Can you work these out from the model? Positions are in its coordinate system, mm. Face numbers are marked on the shaded views. A direction names the side the tool comes from. Round coordinates to 2 decimals unless told otherwise and drop trailing zeros. Loops run counter-clockwise (first coordinate to the right, second up) from the corner with the lowest first, then second, coordinate; pieces in that order, holes last. Notation, with made-up numbers: (50, -28.5) -> (89, -28.5) arc R20 ccw to (89, 10.5) -> close; hole circle Ø9 at (-20.5, 76). An arc over 180 degrees is marked (long way). Answer as a JSON object with one key per item and string values.
```python
from build123d import *

# Parameters (mm, degrees)
SKETCH1_R           = 57.5
BOSS_EXTRUDE1_DEPTH = 18
SKETCH2_R           = 7.5
CUT_EXTRUDE1_DEPTH  = 84.285653026
SKETCH3_R           = 8.629374231
CUT_EXTRUDE2_DEPTH  = 15.116019
CIRPATTERN1_START   = 2.883980854
CIRPATTERN1_DEPTH   = 15.116019146


# Read off the part's stored shape, not the designer's step: CirPattern1
with BuildPart() as part:
    # Sketch1 → Boss-Extrude1 (new body)
    with BuildSketch(Plane(origin=(0, 0, 0), x_dir=(1, 0, 0), z_dir=(0, 1, 0))):
        with Locations(Location((0, 0, 0), (0, 0, 270))):
            Circle(SKETCH1_R)
    extrude(amount=BOSS_EXTRUDE1_DEPTH)

    # Sketch2 → Cut-Extrude1 (cut, through all)
    with BuildSketch(Plane(origin=(0, 0, 0), x_dir=(1, 0, 0), z_dir=(0, 1, 0))):
        with Locations(Location((0, 0, 0), (0, 0, 270))):
            Circle(SKETCH2_R)
    extrude(amount=CUT_EXTRUDE1_DEPTH, mode=Mode.SUBTRACT)

    # Sketch3 → Cut-Extrude2 (cut)
    with BuildSketch(Plane(origin=(0, 18, 0), x_dir=(1, 0, 0), z_dir=(0, 1, 0))):
        with Locations((-14.613023748, 0)):
            Circle(SKETCH3_R)
    extrude(amount=-CUT_EXTRUDE2_DEPTH, mode=Mode.SUBTRACT)

    # CirPattern1 outline → CirPattern1 (cut)
    with BuildSketch(Plane(origin=(0, 0, 0), x_dir=(1, 0, 0), z_dir=(0, 1, 0)).offset(CIRPATTERN1_START)):
        with BuildLine():
            ThreePointArc((7.407428081, -1.174737939), (6.067627458, -4.408389392), (3.406263333, -6.681868758))
            ThreePointArc((3.406263333, -6.681868758), (3.192838488, -8.567271187), (3.396625904, -10.453739627))
            ThreePointArc((3.396625904, -10.453739627), (2.452655059, -8.807771362), (1.17177899, -7.407896732))
            ThreePointArc((1.17177899, -7.407896732), (-2.317627458, -7.132923872), (-5.302241566, -5.30435994))
            ThreePointArc((-5.302241566, -5.30435994), (-7.161317736, -5.684002242), (-8.892482064, -6.460766399))
            ThreePointArc((-8.892482064, -6.460766399), (-9.540804839, -6.981310404), (-10.236214362, -7.43704506))
            ThreePointArc((-10.236214362, -7.43704506), (-7.182295966, -22.104834053), (3.90988597, -12.033391683))
            ThreePointArc((3.90988597, -12.033391683), (18.803494956, -13.661538761), (12.652656784, 0))
            ThreePointArc((12.652656784, 0), (18.803494956, 13.661538761), (3.90988597, 12.033391683))
            ThreePointArc((3.90988597, 12.033391683), (-7.182295966, 22.104834053), (-10.236214362, 7.43704506))
            ThreePointArc((-10.236214362, 7.43704506), (-9.540804839, 6.981310404), (-8.892482064, 6.460766399))
            ThreePointArc((-8.892482064, 6.460766399), (-7.161317736, 5.684002242), (-5.302241566, 5.30435994))
            ThreePointArc((-5.302241566, 5.30435994), (-2.317627458, 7.132923872), (1.17177899, 7.407896732))
            ThreePointArc((1.17177899, 7.407896732), (2.452655059, 8.807771362), (3.396625904, 10.453739627))
            ThreePointArc((3.396625904, 10.453739627), (3.192838488, 8.567271187), (3.406263333, 6.681868758))
            ThreePointArc((3.406263333, 6.681868758), (6.067627458, 4.408389392), (7.407428081, 1.174737939))
            ThreePointArc((7.407428081, 1.174737939), (9.134600443, 0.389137457), (10.99171232, 0))
            ThreePointArc((10.99171232, 0), (9.134600443, -0.389137457), (7.407428081, -1.174737939))
        make_face()
    extrude(amount=CIRPATTERN1_DEPTH, mode=Mode.SUBTRACT)


solid = part.part
```
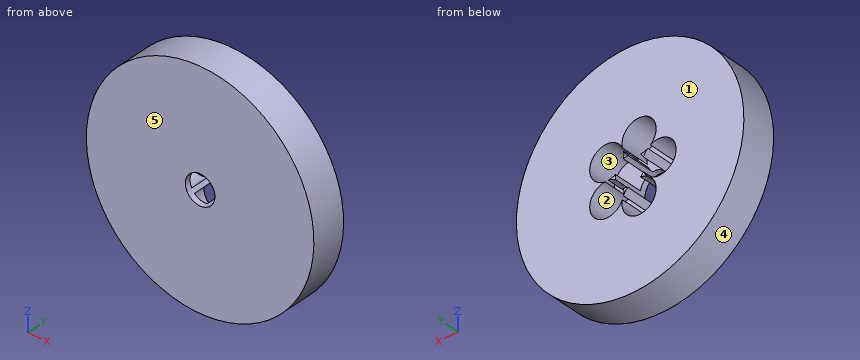
Q1. I want a section at C-C, the plane z = 35.5. Write out the boundary of the cut face in (x, y).
Determined:
{"outline": "(-45.23, 0) -> (45.23, 0) -> (45.23, 18) -> (-45.23, 18) -> close"}
Q2. If I drill on L1, parallel to X at y = 12.5, z = 1; L2, parallel to Z at x = -4.5, y = 5; L3, parallel to Z at x = 14.5, y = 12.5, over which ranges is the centre line in solid material (lowest first)? Write a range as [from, to].
Determined:
{"L1": "[-57.49, -23.18], [7.43, 7.72], [15.93, 57.49]", "L2": "[-57.32, -22.53], [22.53, 57.32]", "L3": "[-55.64, -16.79], [-0.39, 0.39], [16.79, 55.64]"}
Q3. On a 3-axis mill with a long thin cutter (end or side, diameter ignored), from which of +Z, -Z, +X, -X, +Y, -Y can I reach the whole of each face in a straight line? I mean the marked faces 1 and 2. Say none if no direction works.
Determined:
{"face 1": "+Z, -Z, +X, -X, +Y", "face 2": "+Y"}
Q4. I want a section at D-D, the plane z = -44. Write out the boundary of the cut face in (x, y), then the cut area to 3 significant figures.
Determined:
{"outline": "(-37.02, 0) -> (37.02, 0) -> (37.02, 18) -> (-37.02, 18) -> close", "area": "1,330 mm²"}
Q5. We'd pull the mould along Z, two halves only. Please class the marked faces 3, 4 and 5: pulls with the +Z half, pulls with the -Z half, needs draft (parallel to the pull), parting line crosses it, or undercut.
Determined:
{"face 3": "undercut", "face 4": "parting line crosses it", "face 5": "needs draft"}
Q6. I'm going to push flat-ended pins straight in: pin 1 (20 mm diameter, centred on x = -14.61, z = 0, fed in from +Y); pin 2 (1 mm diameter, centred on y = 5, z = 39.5, fed in from +X); pin 3 (13 mm diameter, centred on x = -14.5, z = -1, fed in from +Y); pin 4 (2 mm diameter, centred on x = -30.5, y = 2, fed in from +Z). Where does each tip first touch, or does it pass through?
Determined:
{"pin 1": "y = 18", "pin 2": "x = 42.25", "pin 3": "y = 2.88", "pin 4": "z = 49.36"}
Q7. I want a section at A-A, the plane y = 8.25. Write out the boundary of the cut face in (x, z).
Determined:
{"outline": "circle Ø115 at (0, 0); (-8.89, -6.46) arc R8.63 cw to (-5.3, -5.3) arc R7.5 cw to (-6.68, -3.4) arc R8.63 cw to start; (-8.89, 6.46) arc R8.63 cw to (-6.68, 3.4) arc R7.5 cw to (-5.3, 5.3) arc R8.63 cw to start; (1.17, -7.41) arc R8.63 cw to (3.4, -10.45) arc R8.63 cw to (3.41, -6.68) arc R7.5 cw to start; (1.17, 7.41) arc R7.5 cw to (3.41, 6.68) arc R8.63 cw to (3.4, 10.45) arc R8.63 cw to start; (7.41, -1.17) arc R8.63 cw to (10.99, 0) arc R8.63 cw to (7.41, 1.17) arc R7.5 cw to start; hole (-10.24, -7.44) arc R8.63 ccw (long way) to (3.91, -12.03) arc R8.63 ccw (long way) to (12.65, 0) arc R8.63 ccw (long way) to (3.91, 12.03) arc R8.63 ccw (long way) to (-10.24, 7.44) arc R8.63 ccw (long way) to start"}
Q8. I want a section at B-B, the plane x = -2. Write out the boundary of the cut face in (y, z), then the cut area to 3 significant figures.
Determined:
{"outline": "(0, -57.47) -> (18, -57.47) -> (18, -22.15) -> (2.88, -22.15) -> (2.88, -7.23) -> (0, -7.23) -> close; (0, 7.23) -> (2.88, 7.23) -> (2.88, 22.15) -> (18, 22.15) -> (18, 57.47) -> (0, 57.47) -> close", "area": "1,360 mm²"}
